from build123d import *

# Parameters (mm, degrees)
F1_DEPTH  = 10
F2_R      = 5
F3_DEPTH  = 10.001
F2_R_2    = 15
F4_DEPTH  = 20
F4_FACE_R = 15
F5_DEPTH  = 5


with BuildPart() as f1:
    # F0 (on Top) → F1 (new body)
    with BuildSketch(Plane.XY):
        with BuildLine():
            Line((47.974863, -9.547261), (46.469416, -9.891452))
            ThreePointArc((46.469416, -9.891452), (47.228793, -9.74846), (47.974863, -9.547261))
        make_face()
        with BuildLine():
            Line((4.561589, -19.472851), (46.469416, -9.891452))
            Line((46.469416, -9.891452), (47.974863, -9.547261))
            ThreePointArc((47.974863, -9.547261), (55, 0), (47.974863, 9.547261))
            Line((47.974863, 9.547261), (46.469416, 9.891452))
            Line((46.469416, 9.891452), (4.561589, 19.472851))
            ThreePointArc((4.561589, 19.472851), (0, 20), (-4.561589, 19.472851))
            Line((-4.561589, 19.472851), (-46.469416, 9.891452))
            Line((-46.469416, 9.891452), (-47.974863, 9.547261))
            ThreePointArc((-47.974863, 9.547261), (-55, 0), (-47.974863, -9.547261))
            Line((-47.974863, -9.547261), (-46.469416, -9.891452))
            Line((-46.469416, -9.891452), (-4.561589, -19.472851))
            ThreePointArc((-4.561589, -19.472851), (0, -20), (4.561589, -19.472851))
        make_face()
        with BuildLine():
            Line((46.469416, 9.891452), (47.974863, 9.547261))
            ThreePointArc((47.974863, 9.547261), (47.228793, 9.74846), (46.469416, 9.891452))
        make_face()
        with BuildLine():
            ThreePointArc((-47.974863, -9.547261), (-47.228793, -9.74846), (-46.469416, -9.891452))
            Line((-46.469416, -9.891452), (-47.974863, -9.547261))
        make_face()
        with BuildLine():
            ThreePointArc((-46.469416, 9.891452), (-47.228793, 9.74846), (-47.974863, 9.547261))
            Line((-47.974863, 9.547261), (-46.469416, 9.891452))
        make_face()
    extrude(amount=F1_DEPTH)

    # F2 (on face) → F3 (cut, through all)
    with BuildSketch(Plane.XY.offset(10)):
        with Locations((-40, 0)):
            Circle(F2_R)
        with Locations((40, 0)):
            Circle(F2_R)
    extrude(amount=-F3_DEPTH, mode=Mode.SUBTRACT)

    # F2 (on face) → F4 (join)
    with BuildSketch(Plane.XY.offset(10)):
        with BuildLine():
            ThreePointArc((4.561589, -19.472851), (15.672137, -12.42514), (20, 0))
            ThreePointArc((20, 0), (15.672137, 12.42514), (4.561589, 19.472851))
            ThreePointArc((4.561589, 19.472851), (0, 20), (-4.561589, 19.472851))
            ThreePointArc((-4.561589, 19.472851), (-20, 0), (-4.561589, -19.472851))
            ThreePointArc((-4.561589, -19.472851), (0, -20), (4.561589, -19.472851))
        make_face()
        Circle(F2_R_2, mode=Mode.SUBTRACT)
    extrude(amount=F4_DEPTH)

    # F4_face (on face) → F5 (cut, symmetric)
    with BuildSketch(Plane.XY.offset(10)):
        Circle(F4_FACE_R)
    extrude(amount=F5_DEPTH, both=True, mode=Mode.SUBTRACT)


solid = f1.part
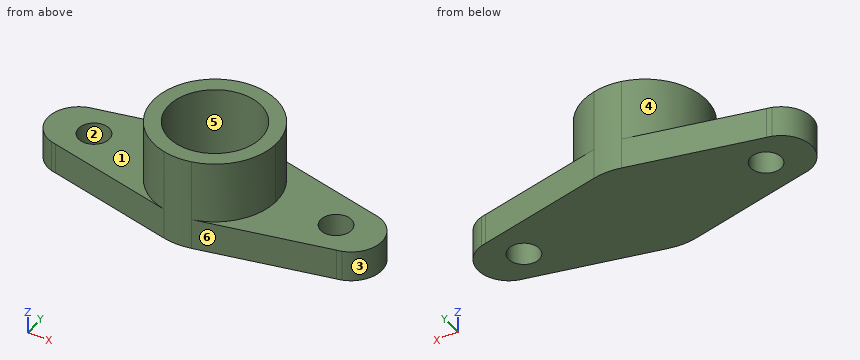
Design review of the part built by this model. Coordinates are the model's own, in mm. Face numbers are marked on the shaded views. A direction names the side the tool comes from. Give positions to 0.01 mm unless a question says otherwise; leave off trailing zeros. Write each loop counter-clockwise with the first axis right and the second up, starting at its lowest first coordinate (ties: lowest second). Pieces come first, ordered by that corner, then holes. Notation, with made-up numbers: M -0.5,32 L 43.5,32 A32 ccw 43.5,67 Z; hole C 14.5,-32 d9. An arc over 180 degrees is marked long. Answer as a JSON object with one key per item and string values. Group by question number.
1) We need section B-B (x = -40.5). Give the boundary of the cut face in (y, z), and give its area (3 significant figures).
2) We need section C-C (y = -1.5). Give the boundary of the cut face in (x, z), and give its area (3 significant figures).
3) We need section A-A (z = 6.25). Give the boundary of the cut face in (x, y).
4) We need section D-D (z = 26.5). Give the boundary of the cut face in (x, y), and give its area (3 significant figures).
5) Mouldability with a two-part tool opening along X and no side actions: class the marked faces 1, 2 and 3 as released by +X, released by -X, zero draft, split by the parting line, or undercut.
6) For line 1 along X through (y, z) = (2.5, 6.5); line 2 along Z through (x, y) = (-4, 13); line 3 along Z through (x, y) = (44, -3.5), list the stretches that pass through material, from the lowest coordinate up.
7) Tool access review of the marked faces 4, 5 and 6: name each direction out of +Z, -Z, +X, -X, +Y, -Y from which nothing blocks a thin tool from reaching the whole face with its end or side.
8) Clearance check with flat-ended pins moving along their axes: pin 1 Ø3 at (y, z) = (-8.5, 25) entering from -X (3 decimals); pin 2 Ø11.5 at (x, y) = (42, 5.5) entering from +Z; pin 3 Ø2 at (x, z) = (34.5, 6) entering from +Y; pin 4 Ø6 at (x, y) = (40, 0) entering from +Z. State where each tip first meets the part, or that it passes through.
Answer key:
{
 "1": {"outline": "M -11.26,0 L -4.97,0 L -4.97,10 L -11.26,10 Z; M 4.97,0 L 11.26,0 L 11.26,10 L 4.97,10 Z", "area": "126 mm²"},
 "2": {"outline": "M -54.89,0 L -44.77,0 L -44.77,10 L -54.89,10 Z; M -35.23,0 L 35.23,0 L 35.23,10 L 19.94,10 L 19.94,30 L 14.92,30 L 14.92,5 L -14.92,5 L -14.92,30 L -19.94,30 L -19.94,10 L -35.23,10 Z; M 44.77,0 L 54.89,0 L 54.89,10 L 44.77,10 Z", "area": "958 mm²"},
 "3": {"outline": "M -47.97,-9.55 A10 ccw -46.47,-9.89 L -4.56,-19.47 A20 ccw 4.56,-19.47 L 46.47,-9.89 A10 ccw 47.97,-9.55 A10 ccw 47.97,9.55 A10 ccw 46.47,9.89 L 4.56,19.47 A20 ccw -4.56,19.47 L -46.47,9.89 A10 ccw -47.97,9.55 A10 ccw Z; hole C -40,0 d10; hole C 0,0 d30; hole C 40,0 d10"},
 "4": {"outline": "M -4.56,-19.47 A20 ccw 4.56,-19.47 A20 ccw 20,0 A20 ccw 4.56,19.47 A20 ccw -4.56,19.47 A20 ccw Z; hole C 0,0 d30", "area": "550 mm²"},
 "5": {"face 1": "zero draft", "face 2": "undercut", "face 3": "released by +X"},
 "6": {"line 1": "x = -54.68 to -44.33, -35.67 to -14.79, 14.79 to 35.67, 44.33 to 54.68", "line 2": "z = 0 to 5", "line 3": "z = 0 to 10"},
 "7": {"face 4": "+Z, -X", "face 5": "+Z", "face 6": "+Z, -Z, +X, -Y"},
 "8": {"pin 1": "stops at x = -18.735", "pin 2": "stops at z = 10", "pin 3": "stops at y = 12.86", "pin 4": "passes through"}
}
